Can you work these out from the drawing? Everything is in mm from the part's minimum corner. A direction names the side the tool comes from. Round coordinates to 2 decimals unless told otherwise and drop trailing zeros. Loops run counter-clockwise (first coordinate to the right, second up) from the corner with the lowest first, then second, coordinate; pieces in that order, holes last. Notation, with made-up numbers: (-26.75, 77) - (-9.75, 77) arc R21 ccw to (-9.75, 102) - close; hole circle Ø10 at (57, 40). An arc over 180 degrees is marked (long way). Answer as a JSON object with one key per item and string values. Group by question number.
1) I want a section at A-A, the plane y = 80. Please give me the cut outline in (x, z).
2) If we mould it in two halves opening along Y, with no side actions, what happens to the marked faces 1, 2 and 3? For each: pulls with the +Y half, pulls with the -Y half, needs draft (parallel to the pull), parting line crosses it, or undercut.
3) If I drill on line 1 along X through (y, z) = (4.5, 6.5); line 2 along Y through (x, z) = (87.25, 9.5); line 3 along Y through (x, z) = (46, 24.75), over which ranges is the centre line in solid material (lowest first)? Write a range as [from, to].
4) Which directions (+Z, -Z, +X, -X, +Y, -Y) give clear straight access to the entire face, cutting with the end or side of a thin tool? Please do the marked faces 4 and 5.
5) I want a section at B-B, the plane x = 82. Please give me the cut outline in (y, z), then the cut area to 3 significant figures.
6) Will this pin go through, and if not, where does the flat tip stop? P1, Ø1.5, axis at x = 67.5, y = 46.5, coming from the +Z side.
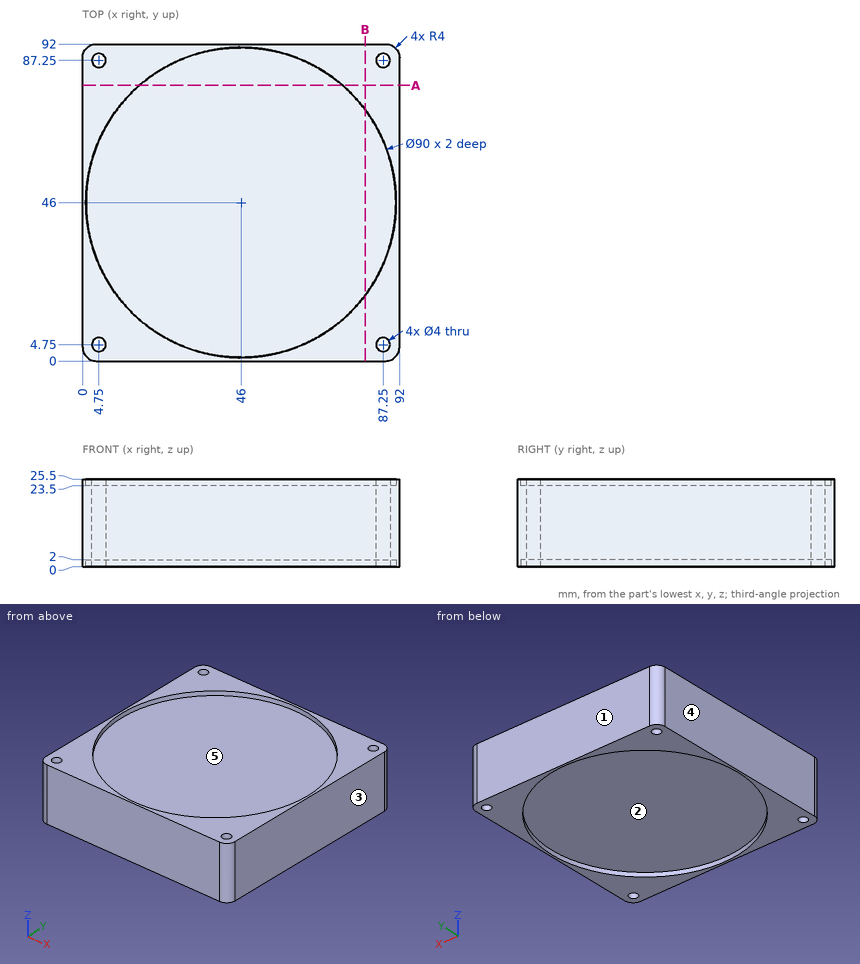
Outcome:
{
 "1": {"outline": "(0, 0) - (16.52, 0) - (16.52, 2) - (75.48, 2) - (75.48, 0) - (92, 0) - (92, 25.5) - (75.48, 25.5) - (75.48, 23.5) - (16.52, 23.5) - (16.52, 25.5) - (0, 25.5) - close"},
 "2": {"face 1": "pulls with the +Y half", "face 2": "undercut", "face 3": "needs draft"},
 "3": {"line 1": "[0, 2.77], [6.73, 85.27], [89.23, 92]", "line 2": "[0, 2.75], [6.75, 85.25], [89.25, 92]", "line 3": "[0, 1], [91, 92]"},
 "4": {"face 4": "+Z, -Z, -X, +Y, -Y", "face 5": "+Z"},
 "5": {"outline": "(0, 0) - (19, 0) - (19, 2) - (73, 2) - (73, 0) - (92, 0) - (92, 25.5) - (73, 25.5) - (73, 23.5) - (19, 23.5) - (19, 25.5) - (0, 25.5) - close", "area": "2,130 mm^2"},
 "6": {"P1": "z = 23.5"}
}
